Source: three-view drawing plus pictorial views. Frame: mm from the lowest corner of the part. Give positions to 0.01 mm unless a question says otherwise; leave off trailing zeros. Write each loop counter-clockwise with the first axis right and the second up, starting at its lowest first coordinate (ties: lowest second). Pieces come first, ordered by that corner, then holes. Notation, with made-up numbers: (-1, 1.5) -> (26, 1.5) arc R22 cw to (26, 33.5) -> close; hole circle Ø8 at (-20, 89.5). An arc over 180 degrees is marked (long way). Answer in a Markdown table with one row per item. Add a question column.
Item 1: Section query C-C on y = 0.2. Output: boundary loops of the cut face in (x, z).
Item 2: Material intervals for probe 1 along X at (y, z) = (0.4, 3); probe 2 along Z at (x, y) = (3, 0.2), sorted ascending. Write a range as from..to.
Item 3: Section query A-A on z = 3. Output: boundary loops of the cut face in (x, y).
Item 4: First-contact query: P1, Ø3, axis at x = 37, z = 16, coming from the -Y side. Flat tip, straight axial feed; report the tip coordinate or a pass-through.
Item 5: Section query B-B on x = 37. Output: boundary loops of the cut face in (y, z).
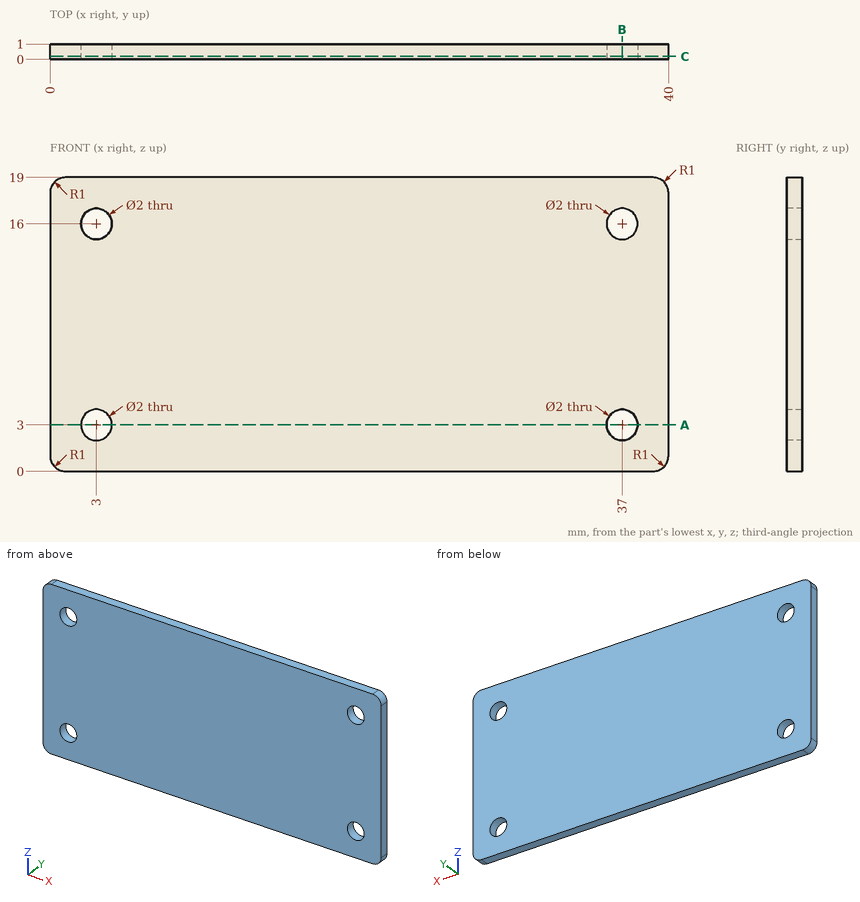
Findings below:
| question | item | result |
|---|---|---|
| 1 | outline | (0, 1) arc R1 ccw to (1, 0) -> (39, 0) arc R1 ccw to (40, 1) -> (40, 18) arc R1 ccw to (39, 19) -> (1, 19) arc R1 ccw to (0, 18) -> close; hole circle Ø2 at (3, 3); hole circle Ø2 at (3, 16); hole circle Ø2 at (37, 3); hole circle Ø2 at (37, 16) |
| 2 | probe 1 | x = 0..2, 4..36, 38..40 |
| 2 | probe 2 | z = 0..2, 4..15, 17..19 |
| 3 | outline | (0, 0) -> (2, 0) -> (2, 1) -> (0, 1) -> close; (4, 0) -> (36, 0) -> (36, 1) -> (4, 1) -> close; (38, 0) -> (40, 0) -> (40, 1) -> (38, 1) -> close |
| 4 | P1 | stops at y = 0 |
| 5 | outline | (0, 0) -> (1, 0) -> (1, 2) -> (0, 2) -> close; (0, 4) -> (1, 4) -> (1, 15) -> (0, 15) -> close; (0, 17) -> (1, 17) -> (1, 19) -> (0, 19) -> close |
